Here's how the part is built. I have some questions about the finished solid (model axes, mm). Face numbers are marked on the shaded views. Give positions to 0.01 mm unless a question says otherwise; leave off trailing zeros. Write each loop counter-clockwise with the first axis right and the second up, starting at its lowest first coordinate (ties: lowest second). Pieces come first, ordered by that corner, then holes. Notation, with made-up numbers: (80, -11.75) - (135, -11.75) arc R15 ccw to (135, 7.25) - close; hole circle Ø5 at (73, -38.5). An arc over 180 degrees is marked (long way). One line per item, written item: value. Start each with the question number.
1) I'm going to push flat-ended pins straight in: P1, Ø4, axis at y = 15.5, z = -1, coming from the -X side; P2, Ø1.7, axis at y = -1, z = -10.5, coming from the +X side; P3, Ø8, axis at x = -7.5, z = 6, coming from the +Y side. Where does each tip first touch, or does it pass through?
2) Imagine slicing it at C-C on y = 4. Write out the boundary of the cut face in (x, z), plus the area to 3 significant figures.
3) Imagine slicing it at D-D on z = 2.5. Write out the boundary of the cut face in (x, y) (3 decimals), plus the area to 3 significant figures.
4) We'd pull the mould along X, two halves only. Please class the marked faces 1, 2 and 3: +X half, -X half, draft (parallel to the pull), parting line (faces both ways), or undercut.
5) Please list where these lines run through material, in increasing order: L1, parallel to Z at x = -0.25, y = -0.25; L2, parallel to Y at x = 0, z = 10; L3, parallel to Z at x = 0, y = 22.25. Write a range as [from, to].
6) Imagine slicing it at B-B on z = 9.25. Write out the boundary of the cut face in (x, y), plus the area to 3 significant figures.
7) Imagine slicing it at A-A on x = 0. Write out the boundary of the cut face in (y, z) (3 decimals), plus the area to 3 significant figures.
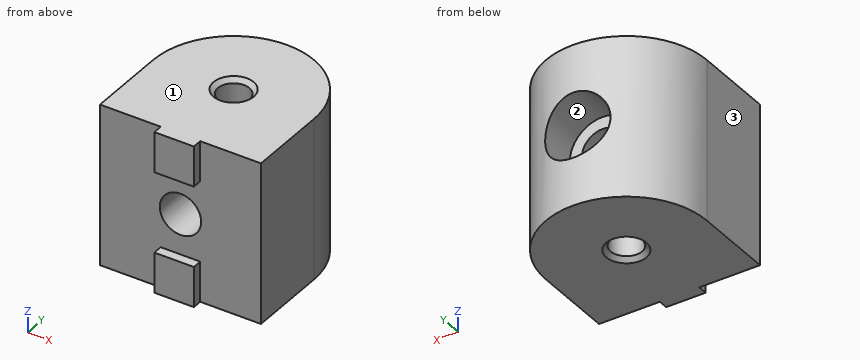
Autodesk Inventor part; units mm, degrees
ref_plane "nub_XY" through (0, 12.7, 12.7) normal (0, 0, 1) x (1, 0, 0)
ref_plane "nub_YZ" through (0, 12.7, 12.7) normal (1, 0, 0) x (0, 1, 0)
ref_plane "nub_ZX" through (0, 12.7, 12.7) normal (0, 1, 0) x (0, 0, 1)
sketch "Sketch_1" plane through (0, 0, 0) normal (0, 0, 1) x (1, 0, 0)
  line L0 (-12.7, 0) -> (12.7, 0)
  line L1 (12.7, 0) -> (12.7, 12.7)
  arc A0 (12.7, 12.7) -> (-12.7, 12.7) centre (0, 12.7) ccw
  line L2 (-12.7, 12.7) -> (-12.7, 0)
extrude "Extrusion1" add sketch "Sketch_1" along normal mid plane 25.4
sketch "Sketch_7" plane through (0, 0, 12.7) normal (0, 0, 1) x (1, 0, 0)
  line L0 (-3.1115, -1.524) -> (3.1115, -1.524)
  line L1 (3.1115, -1.524) -> (3.1115, 0)
  line L2 (3.1115, 0) -> (-3.1115, 0)
  line L3 (-3.1115, 0) -> (-3.1115, -1.524)
extrude "Extrusion2" add sketch "Sketch_7" against normal blind 6.35
sketch "Sketch_2" plane through (0, 0, -12.7) normal (0, 0, 1) x (1, 0, 0)
  line L0 (-3.1115, -1.524) -> (3.1115, -1.524)
  line L1 (3.1115, -1.524) -> (3.1115, 0)
  line L2 (3.1115, 0) -> (-3.1115, 0)
  line L3 (-3.1115, 0) -> (-3.1115, -1.524)
extrude "Extrusion3" add sketch "Sketch_2" along normal blind 6.35
sketch "Sketch_3" plane through (0, 0, 0) normal (1, 0, 0) x (0, 1, 0)
  line L0 (12.7, -12.7) -> (12.7, 12.7)
  line L1 (12.7, 12.7) -> (15.875, 12.7)
  line L2 (15.875, 12.7) -> (15.1879, 12.0129)
  line L3 (15.1879, 12.0129) -> (15.1879, -12.0129)
  line L4 (15.1879, -12.0129) -> (15.875, -12.7)
  line L5 (15.875, -12.7) -> (12.7, -12.7)
  line L6 (12.7, -12.7) -> (12.7, 12.7)
revolve "Revolution1" cut sketch "Sketch_3" angle 360 about axis through (0, 12.7, -12.7) along (0, 0, -1)
thread "Thread1"
sketch "Sketch_4" plane through (0, 0, 0) normal (0, 0, 1) x (1, 0, 0)
  line L0 (0, 0) -> (0, 25.4)
  line L1 (0, 25.4) -> (5.1562, 25.4)
  line L2 (5.1562, 25.4) -> (5.1562, 18.415)
  line L3 (5.1562, 18.415) -> (3.2639, 18.415)
  line L4 (3.2639, 18.415) -> (3.2639, 0)
  line L5 (3.2639, 0) -> (0, 0)
  line L6 (0, 0) -> (0, 25.4)
revolve "Revolution2" cut sketch "Sketch_4" angle 360 about axis through (0, 0, 0) along (0, -1, 0)
ref_plane "nub_XY" through (0, 12.7, 12.7) normal (0, 0, 1) x (1, 0, 0)
ref_plane "nub_YZ" through (0, 12.7, 12.7) normal (1, 0, 0) x (0, 1, 0)
ref_plane "nub_ZX" through (0, 12.7, 12.7) normal (0, 1, 0) x (0, 0, 1)
ref_plane "nub1_XY" through (0, 12.7, -12.7) normal (0, 0, 1) x (1, 0, 0)
ref_plane "nub1_YZ" through (0, 12.7, -12.7) normal (1, 0, 0) x (0, 1, 0)
ref_plane "nub1_ZX" through (0, 12.7, -12.7) normal (0, 1, 0) x (0, 0, 1)
ref_plane "to_dummy_XY" through (0, 0, 0) normal (0, 1, 0) x (1, 0, 0)
ref_plane "to_dummy_YZ" through (0, 0, 0) normal (1, 0, 0) x (0, 0, -1)
ref_plane "to_dummy_ZX" through (0, 0, 0) normal (0, 0, -1) x (0, 1, 0)
ref_plane "to_screw_XY" through (0, 18.415, 0) normal (0, 1, 0) x (1, 0, 0)
ref_plane "to_screw_YZ" through (0, 18.415, 0) normal (1, 0, 0) x (0, 0, -1)
ref_plane "to_screw_ZX" through (0, 18.415, 0) normal (0, 0, -1) x (0, 1, 0)
properties part number "4188_n"
Numbers:
1. P1: x = -12.67
1. P2: x = 3.11
1. P3: y = 24.91
2. outline: (-12.7, -12.7) - (12.7, -12.7) - (12.7, 12.7) - (-12.7, 12.7) - close; hole circle Ø6.53 at (0, 0)
2. area: 612 mm^2
3. outline: (-12.7, 0) - (-2.098, 0) - (-2.098, 11.363) arc R2.488 cw to (-2.098, 14.037) - (-2.098, 18.415) - (-4.51, 18.415) - (-4.51, 24.572) arc R12.7 ccw to (-12.7, 12.7) - close; (2.098, 0) - (12.7, 0) - (12.7, 12.7) arc R12.7 ccw to (4.51, 24.572) - (4.51, 18.415) - (2.098, 18.415) - (2.098, 14.037) arc R2.488 cw to (2.098, 11.363) - close
3. area: 437 mm^2
4. face 1: draft
4. face 2: undercut
4. face 3: -X half
5. L1: [-12.7, -6.35], [6.35, 12.7]
5. L2: [-1.52, 10.21], [15.19, 25.4]
5. L3: [-12.7, -5.16], [5.16, 12.7]
6. outline: (-12.7, 0) - (-3.11, 0) - (-3.11, -1.52) - (3.11, -1.52) - (3.11, 0) - (12.7, 0) - (12.7, 12.7) arc R12.7 ccw to (-12.7, 12.7) - close; hole circle Ø4.98 at (0, 12.7)
6. area: 566 mm^2
7. outline: (-1.524, -12.7) - (9.525, -12.7) - (10.212, -12.013) - (10.212, -3.264) - (0, -3.264) - (0, -6.35) - (-1.524, -6.35) - close; (-1.524, 6.35) - (0, 6.35) - (0, 3.264) - (10.212, 3.264) - (10.212, 12.013) - (9.525, 12.7) - (-1.524, 12.7) - close; (15.188, -12.013) - (15.875, -12.7) - (25.4, -12.7) - (25.4, -5.156) - (18.415, -5.156) - (18.415, -3.264) - (15.188, -3.264) - close; (15.188, 3.264) - (18.415, 3.264) - (18.415, 5.156) - (25.4, 5.156) - (25.4, 12.7) - (15.875, 12.7) - (15.188, 12.013) - close
7. area: 377 mm^2
